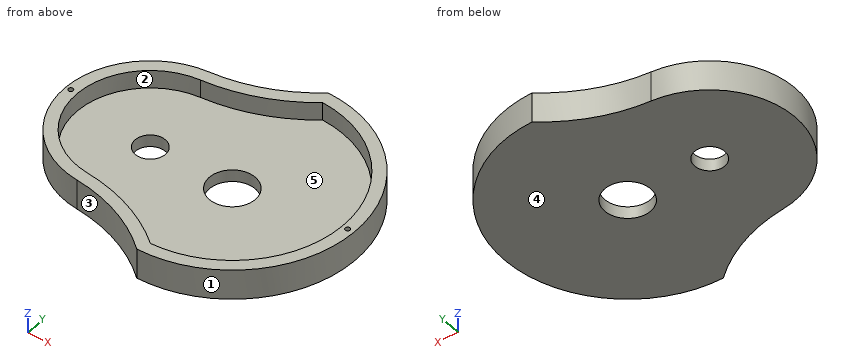
```python
from build123d import *

# Parameters (mm, degrees)
BOSS_EXTRUDE1_DEPTH = 6.35
SHELL1_T            = -2.54
SKETCH3_R           = 4.826
SKETCH3_R_2         = 3.175
CUT_EXTRUDE1_DEPTH  = 2.54
SKETCH2_R           = 0.508
CUT_EXTRUDE2_DEPTH  = 1.27


with BuildPart() as part:
    # Sketch1 → Boss-Extrude1 (new body)
    with BuildSketch(Plane.XY):
        with BuildLine():
            ThreePointArc((0, -25.92959), (25.92959, 0), (0, 25.92959))
            ThreePointArc((0, 25.92959), (-8.900253562, 20.439501874), (-19.05, 17.921918042))
            ThreePointArc((-19.05, 17.921918042), (-35.45459, 0), (-19.05, -17.921918042))
            ThreePointArc((-19.05, -17.921918042), (-8.900253562, -20.439501874), (0, -25.92959))
        make_face()
    extrude(amount=BOSS_EXTRUDE1_DEPTH)

    # Shell1
    shell1_openings = [part.faces().sort_by_distance(p)[0] for p in [
        (-3.11409352, 0, 6.35),
    ]]
    offset(amount=SHELL1_T, openings=shell1_openings, kind=Kind.INTERSECTION)

    # Sketch3 → Cut-Extrude1 (cut)
    with BuildSketch(Plane.XY.offset(2.54)):
        Circle(SKETCH3_R)
        with Locations((-17.4625, 0)):
            Circle(SKETCH3_R_2)
    extrude(amount=-CUT_EXTRUDE1_DEPTH, mode=Mode.SUBTRACT)

    # Sketch2 → Cut-Extrude2 (cut)
    with BuildSketch(Plane.XY.offset(6.35)):
        with Locations((-34.39268404, 0)):
            Circle(SKETCH2_R)
        with Locations((24.569143143, 0)):
            Circle(SKETCH2_R)
    extrude(amount=-CUT_EXTRUDE2_DEPTH, mode=Mode.SUBTRACT)


solid = part.part
```
Model file for the job. Use its own axes, mm. Face numbers are marked on the shaded views. A direction names the side the tool comes from. Round coordinates to 2 decimals unless told otherwise and drop trailing zeros. Write each loop counter-clockwise with the first axis right and the second up, starting at its lowest first coordinate (ties: lowest second). Pieces come first, ordered by that corner, then holes. Notation, with made-up numbers: (22.5, -38) -> (62.5, -38) arc R21 cw to (62.5, -9) -> close; hole circle Ø9 at (69.5, -16). An arc over 180 degrees is marked (long way). Answer as CSV lines item,"result".
1. Pin check, flat tips, straight feed: pin 1 Ø2 at (x, y) = (-2, -1.5) entering from +Z; pin 2 Ø3 at (y, z) = (-10, 5.5) entering from -X; pin 3 Ø11 at (x, y) = (0, 0) entering from +Z; pin 4 Ø1 at (y, z) = (-19, 3.5) entering from +X. Stop position of each tip, or through.
Resolved:
pin 1,"through"
pin 2,"x = -33.32"
pin 3,"z = 2.54"
pin 4,"x = 18.17"
2. Mould opens along Y. For the marked faces 3, 4 and 5 say: +Y half, -Y half, draft (parallel to the pull), parting line (faces both ways), or undercut.
Resolved:
face 3,"-Y half"
face 4,"draft"
face 5,"undercut"
3. Slice it at D-D, the plane x = -16.5. List the corners of the cut face in (y, z).
Resolved:
outline,"(-18.25, 0) -> (-3.03, 0) -> (-3.03, 2.54) -> (-15.67, 2.54) -> (-15.67, 6.35) -> (-18.25, 6.35) -> close; (3.03, 0) -> (18.25, 0) -> (18.25, 6.35) -> (15.67, 6.35) -> (15.67, 2.54) -> (3.03, 2.54) -> close"
4. Tool access for the marked faces 1 and 2: list every direction of +Z, -Z, +X, -X, +Y, -Y with a clear straight run to the whole face (end or side of a thin tool).
Resolved:
face 1,"+Z, -Z, +X"
face 2,"+Z"
5. Slice it at A-A, the plane x = 4. List the corners of the cut face in (y, z), plus the area to 3 significant figures.
Resolved:
outline,"(-25.62, 0) -> (-2.7, 0) -> (-2.7, 2.54) -> (-23.05, 2.54) -> (-23.05, 6.35) -> (-25.62, 6.35) -> close; (2.7, 0) -> (25.62, 0) -> (25.62, 6.35) -> (23.05, 6.35) -> (23.05, 2.54) -> (2.7, 2.54) -> close"
area,"136 mm²"
6. Slice it at B-B, the plane z = 1.25. State how many separate pieces and enclosed holes the cut face has, plus the area to 3 significant figures.
Resolved:
separate pieces,"1"
enclosed holes,"2"
area,"2,190 mm²"
7. Drill centre lines: line 1 (Z direction, x = -16, y = 6); line 2 (X direction, y = -2.5, z = 1.5); line 3 (Y direction, x = 12.5, z = 2.75). Where is each one in solid material? Low to high.
Resolved:
line 1,"0 to 2.54"
line 2,"-35.28 to -19.42, -15.51 to -4.13, 4.13 to 25.81"
line 3,"-22.72 to -19.77, 19.77 to 22.72"
8. Slice it at C-C, the plane x = -7. List the corners of the cut face in (y, z).
Resolved:
outline,"(-21.31, 0) -> (21.31, 0) -> (21.31, 6.35) -> (18.5, 6.35) -> (18.5, 2.54) -> (-18.5, 2.54) -> (-18.5, 6.35) -> (-21.31, 6.35) -> close"
